Verification items for the finished model (mm, model axes). A direction names the side the tool comes from. Round coordinates to 2 decimals unless told otherwise and drop trailing zeros. Write each loop counter-clockwise with the first axis right and the second up, starting at its lowest first coordinate (ties: lowest second). Pieces come first, ordered by that corner, then holes. Notation, with made-up numbers: (-16.75, 32) -> (9.25, 32) arc R6 cw to (9.25, 41) -> close; hole circle Ø4 at (59, 20). An arc over 180 degrees is marked (long way). Answer as a JSON object with one key per item and string values. Group by question number.
(1) Sectioned sample at A-A on y = -39. Record the cut outline in (x, z), and give its area (3 significant figures).
(2) Draft check along X on faces 3 (the face through (188.303, -20.706, 38.006)), 4 (the face through (110.991, -9.625, 28.648)), 5 (the face through (-11.612, -21, 30)), 6 (the face through (221, -42, 11)). Enter one of: released by +X, released by -X, zero draft, split by the parting line, or undercut.
(3) Gauge pin test, flat ends, axial feed: pin 1 Ø6 at (x, y) = (82, -22) entering from +Z; pin 2 Ø9 at (y, z) = (-18.5, 46.5) entering from -X; pin 3 Ø6 at (x, y) = (140.5, -11) entering from +Z; pin 4 Ø1 at (x, y) = (73, -22) entering from -Z. Record the tip position at first contact, or that the pin passes through.
(4) Sectioned sample at D-D on x = 124. Record the cut outline in (y, z), and give its area (3 significant figures).
(5) Sectioned sample at B-B on y = -16.5. Record the cut outline in (x, z).
(6) Set-up check for faces 1 (the face through (108.6, -32.5, 28.6)), 2 (the face through (9.094, -5.787, 53.822)): record each of +Z, -Z, +X, -X, +Y, -Y from which the full face is reachable in a straight line by a thin tool's end or side.
(7) Scan lines: L1, parallel to Z at x = 20, y = -28.5; L2, parallel to Y at x = 10, z = 56; L3, parallel to Z at x = 171.5, y = -18. Record each from-to range of solid material in increasing order. Write a range as from..to.
(8) Sectioned sample at C-C on z = 58. Record the cut outline in (x, y), and give its area (3 significant figures).
```python
from build123d import *

# Parameters (mm, degrees)
F4_DEPTH = 42
F6_DEPTH = 127
F7_DEPTH = 127
F8_R     = 14.6889125436
F9_DEPTH = 42


# Not quite as in the source:
# - a feature of the source that left no trace in its solid (it failed there, or was rolled back) is left out


with BuildPart() as f4:
    # F2 (on Front) → F4 (new body)
    with BuildSketch(Plane.XZ):
        with BuildLine():
            Line((227.6969850063, 0), (228.1920313835, 19.6573249996))
            ThreePointArc((228.1920313835, 19.6573249996), (175.3476715099, 42.1359663093), (118.6285698173, 51.1225779498))
            Line((118.6285698173, 51.1225779498), (43.1631058455, 75.087800622))
            Line((43.1631058455, 75.087800622), (-11.6123249754, 75.087800622))
            Line((-11.6123249754, 75.087800622), (-11.6123249754, 0))
            Line((-11.6123249754, 0), (227.6969850063, 0))
        make_face()
    extrude(amount=F4_DEPTH)

    # F5 (on face) → F6 (cut)
    with BuildSketch(Plane(origin=(0, 0, 0), x_dir=(1, 0, 0), z_dir=(0, 0, -1))):
        with BuildLine():
            ThreePointArc((214.5471125841, 0), (128.9673938043, 10.0631527668), (43.3876750246, 0))
            Line((43.3876750246, 0), (214.5471125841, 0))
        make_face()
    extrude(amount=-F6_DEPTH, mode=Mode.SUBTRACT)

    # F5 (on face) → F7 (cut)
    with BuildSketch(Plane(origin=(0, 0, 0), x_dir=(1, 0, 0), z_dir=(0, 0, -1))):
        with BuildLine():
            Line((214.5471125841, 42), (43.3876750246, 42))
            ThreePointArc((43.3876750246, 42), (128.9673938043, 31.9368472332), (214.5471125841, 42))
        make_face()
    extrude(amount=-F7_DEPTH, mode=Mode.SUBTRACT)

    # F8 (on face) → F9 (cut)
    with BuildSketch(Plane(origin=(-11.6123249754, 0, 0), x_dir=(0, -1, 0), z_dir=(-1, 0, 0))):
        with Locations((20.4619783908, 53.1766302884)):
            Circle(F8_R)
    extrude(amount=-F9_DEPTH, mode=Mode.SUBTRACT)


solid = f4.part
```
Computed values:
{
 "1": {"outline": "(-11.61, 0) -> (57.12, 0) -> (57.12, 70.65) -> (43.16, 75.09) -> (-11.61, 75.09) -> close; (200.81, 0) -> (227.7, 0) -> (228.19, 19.66) arc R234.93 ccw to (200.81, 33.21) -> close", "area": "5,860 mm2"},
 "2": {"face 3": "released by +X", "face 4": "undercut", "face 5": "released by -X", "face 6": "zero draft"},
 "3": {"pin 1": "z = 63.71", "pin 2": "x = 30.39", "pin 3": "z = 49.71", "pin 4": "z = 0"},
 "4": {"outline": "(-31.97, 0) -> (-10.03, 0) -> (-10.03, 50.88) -> (-31.97, 50.88) -> close", "area": "1,120 mm2"},
 "5": {"outline": "(-11.61, 0) -> (227.7, 0) -> (228.19, 19.66) arc R234.93 ccw to (118.63, 51.12) -> (43.16, 75.09) -> (-11.61, 75.09) -> (-11.61, 67.32) -> (30.39, 67.32) -> (30.39, 39.03) -> (-11.61, 39.03) -> close"},
 "6": {"face 1": "+Z, -Z, -Y", "face 2": "-X"},
 "7": {"L1": "0..40.88, 65.47..75.09", "L2": "-42..-34.88, -6.05..0", "L3": "0..43.21"},
 "8": {"outline": "(-11.61, -42) -> (43.39, -42) arc R368.93 cw to (96.97, -33.33) -> (96.97, -8.67) arc R368.93 cw to (43.39, 0) -> (-11.61, 0) -> (-11.61, -6.59) -> (30.39, -6.59) -> (30.39, -34.34) -> (-11.61, -34.34) -> close", "area": "2,860 mm2"}
}
